For this review, use the dimensioned drawing (mm, ordinates from the lowest corner) and the shaded views. A direction names the side the tool comes from. Coordinates: 2 decimals unless noted, no trailing zeros. Order: outer loops, then holes, each group sorted by start corner. A loop starts at its lowest first (then second) coordinate and runs counter-clockwise, first axis right, second up. Notation, with made-up numbers: M 44.25,85 L 52.25,85 A20 ccw 52.25,115 Z; hole C -30.5,-26.75 d1. An arc over 180 degrees is marked long. Write each question's results on one line, items separated by ' | '.
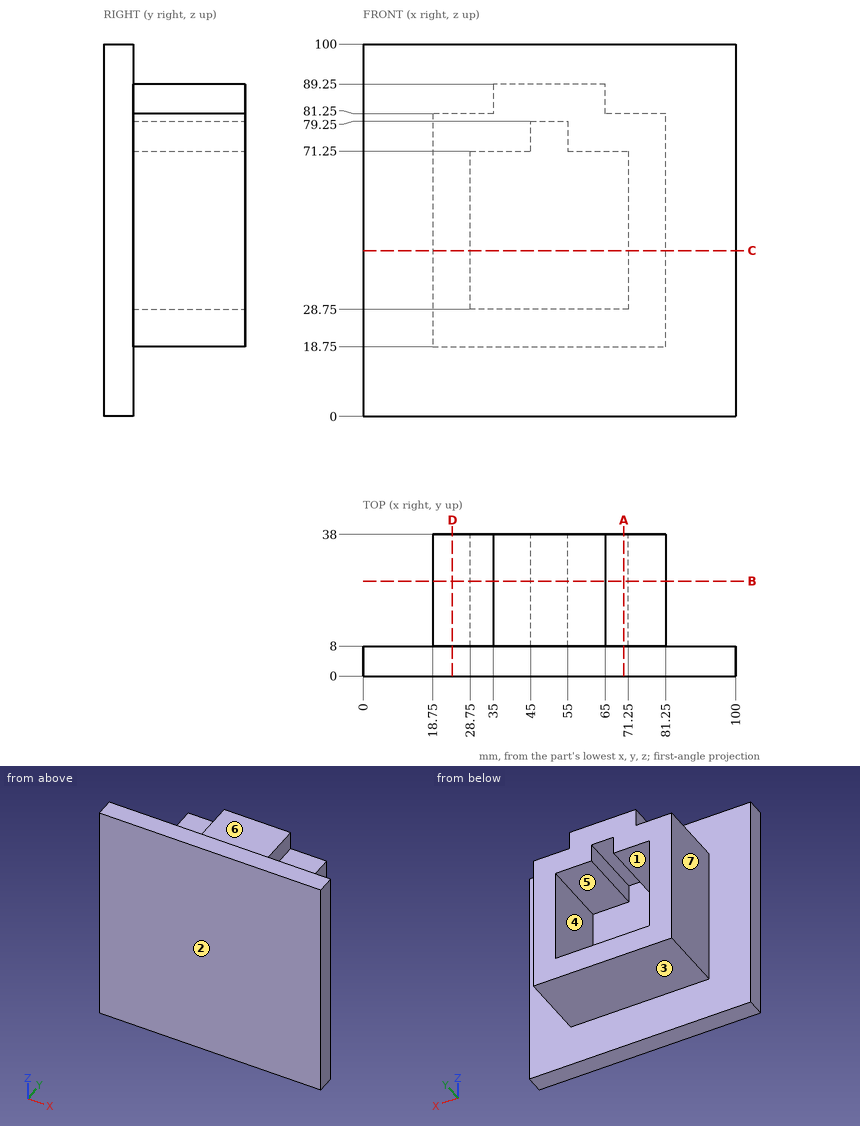
1) Take a section at B-B on y = 25.5. State the section outline as (x, z) points.
Solutions:
outline: M 18.75,18.75 L 81.25,18.75 L 81.25,81.25 L 65,81.25 L 65,89.25 L 35,89.25 L 35,81.25 L 18.75,81.25 Z; hole M 28.75,28.75 L 71.25,28.75 L 71.25,71.25 L 55,71.25 L 55,79.25 L 45,79.25 L 45,71.25 L 28.75,71.25 Z
2) For pin 1 (1.5 mm diameter, centred on y = 20, z = 21, fed in from -X); pin 2 (8 mm diameter, centred on x = 67, y = 23, fed in from -Z); pin 3 (18 mm diameter, centred on x = 70, y = 29, fed in from +Z); pin 4 (10 mm diameter, centred on x = 85.5, z = 33.5, fed in from +Y), all flat-tipped, find the tip position at first contact; note any pin that passes through.
Solutions:
pin 1: x = 18.75 | pin 2: z = 18.75 | pin 3: z = 89.25 | pin 4: y = 38
3) Take a section at C-C on z = 44.5. State the section outline as (x, y) points.
Solutions:
outline: M 0,0 L 100,0 L 100,8 L 81.25,8 L 81.25,38 L 71.25,38 L 71.25,8 L 28.75,8 L 28.75,38 L 18.75,38 L 18.75,8 L 0,8 Z
4) The part is to be moulded in two halves that separate along Z. For the marked faces 4, 5, 6 and 7, say which applies: pulls with the +Z half, pulls with the -Z half, needs draft (parallel to the pull), parting line crosses it, or undercut.
Solutions:
face 4: undercut | face 5: undercut | face 6: pulls with the +Z half | face 7: needs draft
5) For the marked faces 1, 2 and 3, list the 3-axis set-ups (+Z, -Z, +X, -X, +Y, -Y) from which the entire face can be reached by the end or side of a thin tool; tool diameter is ignored.
Solutions:
face 1: +Y | face 2: +Z, -Z, +X, -X, -Y | face 3: -Z, +X, -X, +Y
6) Take a section at A-A on x = 70. State the section outline as (y, z) points.
Solutions:
outline: M 0,0 L 8,0 L 8,18.75 L 38,18.75 L 38,28.75 L 8,28.75 L 8,71.25 L 38,71.25 L 38,81.25 L 8,81.25 L 8,100 L 0,100 Z
7) To check wall thickness, follow line 1 along X through (y, z) = (34.5, 77); line 2 along Z through (x, y) = (48, 16); line 3 along X through (y, z) = (33, 29.5). State the ranges of each line that lie inside material, in increasing order.
Solutions:
line 1: 18.75 to 45, 55 to 81.25 | line 2: 18.75 to 28.75, 79.25 to 89.25 | line 3: 18.75 to 28.75, 71.25 to 81.25
8) Take a section at D-D on x = 24. State the section outline as (y, z) points, plus the area to 4 significant figures.
Solutions:
outline: M 0,0 L 8,0 L 8,18.75 L 38,18.75 L 38,81.25 L 8,81.25 L 8,100 L 0,100 Z | area: 2,675 mm2
